```python
from build123d import *

# Parameters (mm, degrees)
SKETCH_R      = 7.9121
SKETCH_R_2    = 2.667
PAD_DEPTH     = 20.193
SKETCH001_R   = 19.6784
SKETCH001_R_2 = 5.334
PAD001_DEPTH  = 2
SKETCH002_R   = 19.6784
SKETCH002_R_2 = 17.6784
PAD002_DEPTH  = 20.193


with BuildPart() as part:
    # Sketch → Pad (new body)
    with BuildSketch(Plane.XY):
        Circle(SKETCH_R)
        Circle(SKETCH_R_2, mode=Mode.SUBTRACT)
    extrude(amount=PAD_DEPTH)

    # Sketch001 → Pad001 (join)
    with BuildSketch(Plane.XY):
        Circle(SKETCH001_R)
        Circle(SKETCH001_R_2, mode=Mode.SUBTRACT)
    extrude(amount=PAD001_DEPTH)

    # Sketch002 → Pad002 (join)
    with BuildSketch(Plane.XY):
        Circle(SKETCH002_R)
        Circle(SKETCH002_R_2, mode=Mode.SUBTRACT)
    extrude(amount=PAD002_DEPTH)


solid = part.part
```
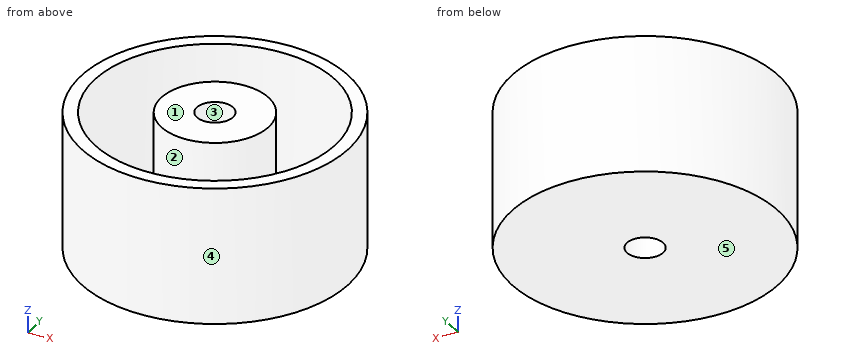
The listing builds one solid part. Answer for the finished solid, in the listing's coordinates (mm). Face numbers are marked on the shaded views. A direction names the side the tool comes from. Give positions to 0.01 mm unless a question says otherwise; leave off trailing zeros. Order: outer loops, then holes, each group sorted by start corner. A loop starts at its lowest first (then second) coordinate and runs counter-clockwise, first axis right, second up. Notation, with made-up numbers: (15.25, 5.5) -> (69.25, 5.5) arc R15 ccw to (69.25, 12.5) -> close; hole circle Ø3 at (67, 25). An arc over 180 degrees is marked (long way). One line per item, written item: value.
1) Find section A-A, the plane z = 7.75. Determine the outline of the cut face in (x, y).
Reported:
outline: circle Ø39.36 at (0, 0); circle Ø15.82 at (0, 0); hole circle Ø35.36 at (0, 0); hole circle Ø5.33 at (0, 0)
2) Find section D-D, the plane x = 4. Determine the outline of the cut face in (y, z), plus the area to 3 significant figures.
Reported:
outline: (-19.27, 0) -> (19.27, 0) -> (19.27, 20.19) -> (17.22, 20.19) -> (17.22, 2) -> (6.83, 2) -> (6.83, 20.19) -> (-6.83, 20.19) -> (-6.83, 2) -> (-17.22, 2) -> (-17.22, 20.19) -> (-19.27, 20.19) -> close
area: 400 mm^2
3) Flat-ended cylindrical pins translate along their axes: P1, Ø4, axis at x = 14, z = 15, coming from the +Y side; P2, Ø12, axis at x = -13.5, z = 13.5, coming from the -Y side; P3, Ø10, axis at y = -15, z = 16.5, coming from the +X side. Find the tip coordinate at first contact, or state that the pin passes through.
Reported:
P1: stops at y = 15.6
P2: stops at y = -18.19
P3: stops at x = 16.95
4) Find section B-B, the plane y = 0. Determine the outline of the cut face in (x, z), plus the area to 3 significant figures.
Reported:
outline: (-19.68, 0) -> (-2.67, 0) -> (-2.67, 20.19) -> (-7.91, 20.19) -> (-7.91, 2) -> (-17.68, 2) -> (-17.68, 20.19) -> (-19.68, 20.19) -> close; (2.67, 0) -> (19.68, 0) -> (19.68, 20.19) -> (17.68, 20.19) -> (17.68, 2) -> (7.91, 2) -> (7.91, 20.19) -> (2.67, 20.19) -> close
area: 332 mm^2
5) Find the intervals of material crossed by line 1 (Y direction, x = 0, z = 10.25); line 2 (Y direction, x = 1, z = 12.25); line 3 (X direction, y = -5.5, z = 14.75), in increasing order.
Reported:
line 1: y = -19.68 to -17.68, -7.91 to -2.67, 2.67 to 7.91, 17.68 to 19.68
line 2: y = -19.65 to -17.65, -7.85 to -2.47, 2.47 to 7.85, 17.65 to 19.65
line 3: x = -18.89 to -16.8, -5.69 to 5.69, 16.8 to 18.89
6) A tool of negligible diameter and unlimited length cuts with its end or side. For the marked faces 1 and 2, from which of +Z, -Z, +X, -X, +Y, -Y can it reach the whole face along a straight path? Write none if from no direction.
Reported:
face 1: +Z, +X, -X, +Y, -Y
face 2: +Z
7) Determine the mould class of the marked faces 3, 4 and 5 for opening direction Y: pulls with the +Y half, pulls with the -Y half, needs draft (parallel to the pull), parting line crosses it, or undercut.
Reported:
face 3: undercut
face 4: parting line crosses it
face 5: needs draft
